```python
from build123d import *

# Parameters (mm, degrees)
F0_W     = 200
F0_H     = 100
F1_DEPTH = 25
F2_R     = 5
F3_R     = 30
F4_DEPTH = 25


with BuildPart() as f1:
    # F0 (on Front) → F1 (new body)
    with BuildSketch(Plane.XZ):
        Rectangle(F0_W, F0_H)
    extrude(amount=F1_DEPTH)

    # F2
    f2_edges = [f1.edges().sort_by_distance(p)[0] for p in [
        (-100, -12.5, -50),
        (100, -12.5, -50),
        (100, -12.5, 50),
        (-100, -12.5, 50),
    ]]
    fillet(f2_edges, radius=F2_R)

    # F3 (on face) → F4 (join)
    with BuildSketch(Plane.XZ.offset(25)):
        Circle(F3_R)
    extrude(amount=F4_DEPTH)


solid = f1.part
```
For this review, take the finished solid that the model builds, in its own axes (mm). A direction names the side the tool comes from. Coordinates: 2 decimals unless noted, no trailing zeros. Write each loop counter-clockwise with the first axis right and the second up, starting at its lowest first coordinate (ties: lowest second). Pieces come first, ordered by that corner, then holes.
(1) Wall thickness on probe 1 along Y at (x, z) = (86.5, 2.5); probe 2 along X at (y, z) = (-28.5, 17); probe 3 along X at (y, z) = (-33, -23): over which ranges is each line inside the solid? List them lowest first.
(2) Add section C-C on y = -39. Give the boundary of the cut face in (x, z).
(3) Add section B-B on x = 0. Give the boundary of the cut face in (y, z).
(4) Tool access review of faces 1 (the face through (-99, -13, -48)), 2 (the face through (-29.97, -37.33, 1.32)): name each direction out of +Z, -Z, +X, -X, +Y, -Y from which nothing blocks a thin tool from reaching the whole face with its end or side.
(5) For pin 1 Ø8 at (x, z) = (-18, 30.5) entering from +Y; pin 2 Ø6 at (x, z) = (-44, 37) entering from -Y; pin 3 Ø1 at (x, y) = (4.5, -30.5) entering from +Z, all flat-tipped, find the tip position at first contact; note any pin that passes through.
(6) Add section A-A on z = 0. Give the boundary of the cut face in (x, y), then the cut area to 3 significant figures.
(7) Add section D-D on x = 52.5. Give the boundary of the cut face in (y, z), then the cut area to 3 significant figures.
Answer sheet:
1. probe 1: y = -25 to 0
1. probe 2: x = -24.72 to 24.72
1. probe 3: x = -19.26 to 19.26
2. outline: circle Ø60 at (0, 0)
3. outline: (-50, -30) - (-25, -30) - (-25, -50) - (0, -50) - (0, 50) - (-25, 50) - (-25, 30) - (-50, 30) - close
4. face 1: -Z, -X, +Y, -Y
4. face 2: -Y
5. pin 1: stops at y = 0
5. pin 2: stops at y = -25
5. pin 3: stops at z = 29.73
6. outline: (-100, -25) - (-30, -25) - (-30, -50) - (30, -50) - (30, -25) - (100, -25) - (100, 0) - (-100, 0) - close
6. area: 6,500 mm2
7. outline: (-25, -50) - (0, -50) - (0, 50) - (-25, 50) - close
7. area: 2,500 mm2
